Geometry check sheet. Reference: the model listing, model coordinates, mm. Round coordinates to 2 decimals unless told otherwise and drop trailing zeros. Write each loop counter-clockwise with the first axis right and the second up, starting at its lowest first coordinate (ties: lowest second). Pieces come first, ordered by that corner, then holes. Notation, with made-up numbers: (18, 4.25) -> (55, 4.25) arc R18 ccw to (55, 33.25) -> close; hole circle Ø7 at (50, -5.75). An arc over 180 degrees is marked (long way). Return JSON: item names as keys, results as strings. Group by question number.
Autodesk Inventor part; units mm, degrees
ref_plane "YZ Plane" through (0, 0, 0) normal (1, 0, 0) x (0, 1, 0)
ref_plane "XZ Plane" through (0, 0, 0) normal (0, 1, 0) x (-1, 0, 0)
ref_plane "XY Plane" through (0, 0, 0) normal (0, 0, 1) x (1, 0, 0)
sketch "Sketch1" plane through (0, 0, 0) normal (0, 0, 1) x (1, 0, 0)
  line L0 (0, 0) -> (107, 0)
  line L1 (107, 0) -> (107, 65)
  line L2 (107, 65) -> (0, 65)
  line L3 (0, 65) -> (0, 0)
  dimension "d0" = 107
  dimension "d1" = 65
extrude "Extrusion1" add sketch "Sketch1" along normal blind 3
sketch "Sketch2" plane through (0, 0, 3) normal (0, 0, 1) x (1, 0, 0)
  line L0 (0, 0) -> (107, 0)
  line L1 (53.5, 0) -> (53.5, 65)
  line L2 (107, 0) -> (107, 26)
  line L3 (107, 0) -> (107, 65)
  line L4 (107, 26) -> (88, 26)
  line L5 (88, 26) -> (88, 38)
  line L6 (88, 38) -> (107, 38)
  line L7 (0, 0) -> (0, 26)
  line L8 (0, 26) -> (19, 26)
  line L9 (19, 26) -> (19, 38)
  line L10 (19, 38) -> (0, 38)
  line L11 (0, 26) -> (0, 38)
  line L12 (0, 65) -> (0, 0)
  dimension "d8" = 26
  dimension "d9" = 19
  dimension "d10" = 12
  dimension "d11" = 19
extrude "Extrusion2" cut sketch "Sketch2" against normal blind 50.975
sketch "Sketch3" plane through (0, 0, 0) normal (0, -1, 0) x (1, 0, 0)
  line L0 (0, 0) -> (0, 3)
  line L1 (0, 1.5) -> (107, 1.5)
  line L2 (107, 0) -> (107, 3)
  line L3 (0, 3) -> (107, 3)
  line L4 (53.5, 3) -> (53.5, 0)
  line L5 (0, 0) -> (107, 0)
  line L6 (53.5, 1.5) -> (43.3165, 1.5)
  line L7 (53.5, 1.5) -> (63.6835, 1.5)
  line L8 (43.3165, 1.5) -> (39.3165, 1.5)
  line L9 (41.3165, 1.5) -> (39.3165, 1.5)
  line L10 (39.3165, 1.5) -> (39.3165, 3)
  line L11 (43.3165, 1.5) -> (43.3165, 0)
  line L12 (39.3165, 3) -> (43.3165, 3)
  line L13 (43.3165, 3) -> (43.3165, 0)
  line L14 (43.3165, 0) -> (39.3165, 0)
  line L15 (39.3165, 0) -> (39.3165, 3)
  line L16 (67.6835, 1.5) -> (67.6835, 3)
  line L17 (67.6835, 3) -> (63.6835, 3)
  line L18 (63.6835, 3) -> (63.6835, 0)
  line L19 (63.6835, 0) -> (67.6835, 0)
  line L20 (67.6835, 0) -> (67.6835, 3)
  line L21 (39.3165, 1.5) -> (18.9495, 1.5)
  line L22 (29.133, 1.5) -> (29.133, 3)
  line L23 (18.9495, 3) -> (14.9495, 3)
  line L24 (14.9495, 3) -> (14.9495, 0)
  line L25 (14.9495, 0) -> (18.9495, 0)
  line L26 (18.9495, 0) -> (18.9495, 3)
  line L27 (88.0505, 0) -> (88.0505, 3)
  line L28 (88.0505, 3) -> (92.0505, 3)
  line L29 (92.0505, 3) -> (92.0505, 0)
  line L30 (92.0505, 0) -> (88.0505, 0)
  point P0 (92.0505, 0)
  point P1 (63.6835, 0)
  point P2 (14.9495, 0)
  dimension "d14" = 10.1835
  dimension "d15" = 10.1835
  dimension "d16" = 4
  dimension "d17" = 2
  dimension "d18" = 1.5
  dimension "d19" = 1.5
  dimension "d20" = 20.367
extrude "Extrusion3" add sketch "Sketch3" along normal blind 2.7 contours L24 L1 L26 L5 | L24 L3 L26 L1 | L15 L1 L11 L5 | L10 L3 L13 L1 | L18 L1 L20 L5 | L18 L3 L16 L1 | L27 L1 L29 L5 | L27 L3 L29 L1
extrude "Extrusion4" add sketch "Sketch3" against normal blind 2.7 from surface at -65 contours L24 L1 L26 L5 | L24 L3 L26 L1 | L15 L1 L11 L5 | L10 L3 L13 L1 | L18 L1 L20 L5 | L18 L3 L16 L1 | L27 L1 L29 L5 | L27 L3 L29 L1
properties part number "carcasa_piezaFrontal"
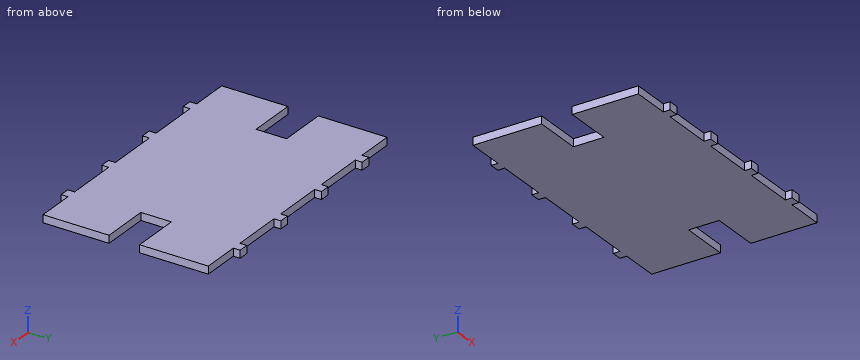
1) Go/stop test with flat-tipped pins: P1, Ø1.4, axis at y = -2, z = 1.5, coming from the -X side; P2, Ø1.4, axis at y = 66.5, z = 1.5, coming from the +X side; P3, Ø1.5, axis at x = 27.5, z = 1.5, coming from the +Y side. Record where each tip stops, or that it passes through.
2) Sectioned sample at A-A on x = 10.5. Enter the section's corners in (y, z), and give its area (3 significant figures).
3) Sectioned sample at B-B on x = 91. Enter the section's corners in (y, z).
4) Sectioned sample at C-C on x = 24. Enter the section's corners in (y, z), and give its area (3 significant figures).
5) Material ranges on probe 1 along Y at (x, z) = (7.5, 2.45); probe 2 along Y at (x, z) = (16, 2.3); probe 3 along Y at (x, z) = (46.5, 1.35), recorded low to high. Write a range as [from, to].
Evaluation:
{
 "1": {"P1": "stops at x = 14.95", "P2": "stops at x = 92.05", "P3": "stops at y = 65"},
 "2": {"outline": "(0, 0) -> (26, 0) -> (26, 3) -> (0, 3) -> close; (38, 0) -> (65, 0) -> (65, 3) -> (38, 3) -> close", "area": "159 mm2"},
 "3": {"outline": "(-2.7, 0) -> (26, 0) -> (26, 3) -> (-2.7, 3) -> close; (38, 0) -> (67.7, 0) -> (67.7, 3) -> (38, 3) -> close"},
 "4": {"outline": "(0, 0) -> (65, 0) -> (65, 3) -> (0, 3) -> close", "area": "195 mm2"},
 "5": {"probe 1": "y = [0, 26], [38, 65]", "probe 2": "y = [-2.7, 26], [38, 67.7]", "probe 3": "y = [0, 65]"}
}
